Job drawing, mm, ordinate dimensions from the low corner. One solid piece. A direction names the side the tool comes from. Round coordinates to 2 decimals unless told otherwise and drop trailing zeros. Loops run counter-clockwise (first coordinate to the right, second up) from the corner with the lowest first, then second, coordinate; pieces in that order, holes last.
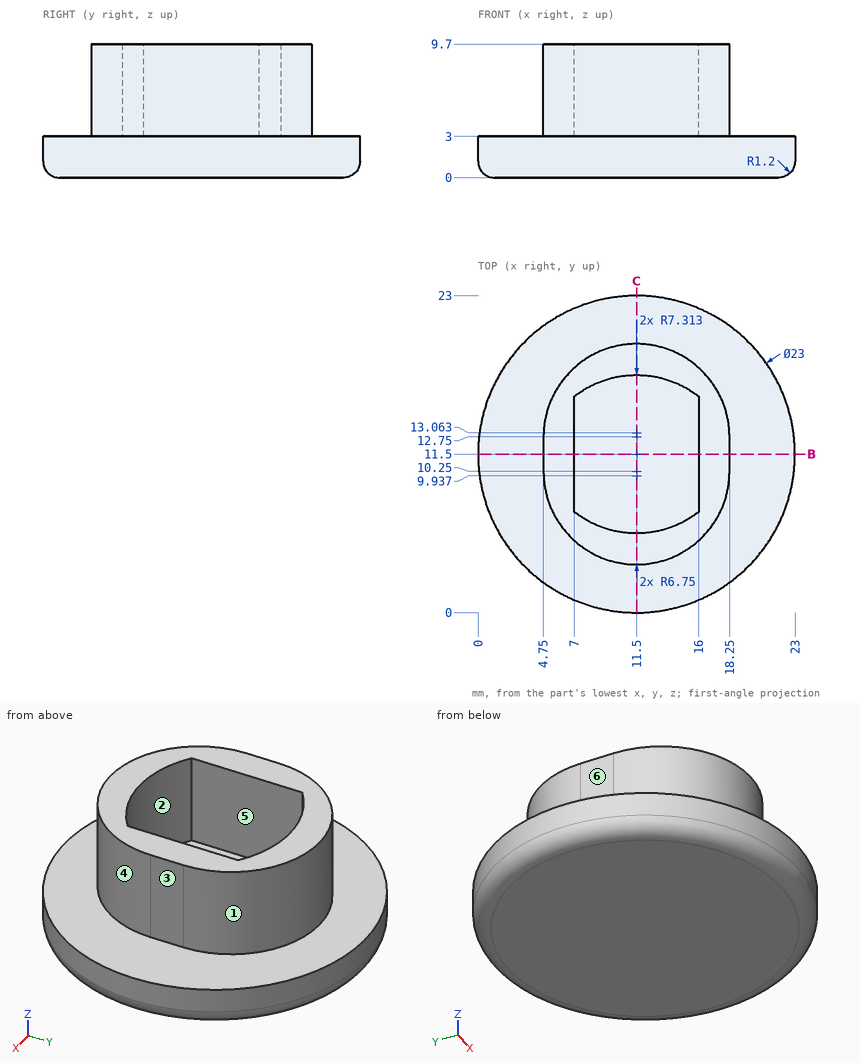
1) Drop flat-ended pins along their axis: pin 1 Ø2 at (y, z) = (11.5, 5) entering from +X; pin 2 Ø2 at (x, z) = (6, 5) entering from -Y; pin 3 Ø3.5 at (y, z) = (12, 7) entering from -X. Give the stop position or say it passes through.
Values:
pin 1: stops at x = 18.25
pin 2: stops at y = 5.22
pin 3: stops at x = 4.75
2) Slice it at B-B, the plane y = 11.5. Give the cut face in (x, z).
Values:
outline: (0, 1.2) arc R1.2 ccw to (1.2, 0) - (21.8, 0) arc R1.2 ccw to (23, 1.2) - (23, 3) - (18.25, 3) - (18.25, 9.7) - (16, 9.7) - (16, 3) - (7, 3) - (7, 9.7) - (4.75, 9.7) - (4.75, 3) - (0, 3) - close
3) Tool access for the marked faces 4, 5 and 6: list every direction of +Z, -Z, +X, -X, +Y, -Y with a clear straight run to the whole face (end or side of a thin tool).
Values:
face 4: +Z, -Y
face 5: +Z
face 6: +Z, -X, +Y, -Y
4) Mould opens along X. For the marked faces 1, 2 and 3 say: released by +X, released by -X, zero draft, split by the parting line, or undercut.
Values:
face 1: split by the parting line
face 2: undercut
face 3: released by +X
5) Wall check: line 1 along X through (y, z) = (11.5, 7.75); line 2 along Y through (x, z) = (15.75, 5) (1 decimal). Give the ranges that are in metal, low to high.
Values:
line 1: x = 4.75 to 7, 16 to 18.25
line 2: y = 5 to 7.1, 15.9 to 18
6) Slice it at C-C, the plane x = 11.5. Give the cut face in (y, z).
Values:
outline: (0, 1.2) arc R1.2 ccw to (1.2, 0) - (21.8, 0) arc R1.2 ccw to (23, 1.2) - (23, 3) - (19.5, 3) - (19.5, 9.7) - (17.25, 9.7) - (17.25, 3) - (5.75, 3) - (5.75, 9.7) - (3.5, 9.7) - (3.5, 3) - (0, 3) - close
